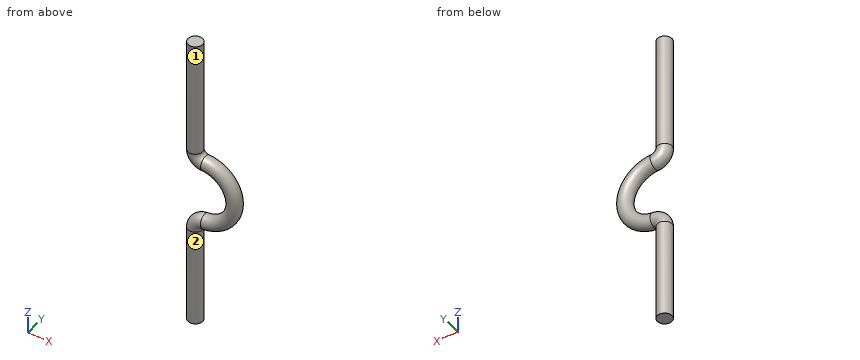
from build123d import *

# Parameters (mm, degrees)
CROQUIS2_R = 3.5


with BuildPart() as part:
    # Barrer2: sweep along a path in Croquis1
    with BuildLine(Plane(origin=(0, 0, 0), x_dir=(1, 0, 0), z_dir=(0, 1, 0))) as barrer2_path:
        Line((0, 0), (0, 55.031280577))
        ThreePointArc((0, 55.031280577), (1.355655066, 58.454546562), (4.6875, 60.021505397))
        ThreePointArc((4.6875, 60.021505397), (18.75, 74.992179856), (4.6875, 89.962854314))
        ThreePointArc((4.6875, 89.962854314), (1.355655066, 91.52981315), (0, 94.953079134))
        Line((0, 94.953079134), (0, 142))
    # Croquis2 → Barrer2 (sweep)
    with BuildSketch(Plane.XY):
        Circle(CROQUIS2_R)
    sweep(path=barrer2_path.line)


solid = part.part
Build history of the part. All positions in model axes, mm. Face numbers are marked on the shaded views. A direction names the side the tool comes from. Round coordinates to 2 decimals unless told otherwise and drop trailing zeros. Write each loop counter-clockwise with the first axis right and the second up, starting at its lowest first coordinate (ties: lowest second). Pieces come first, ordered by that corner, then holes. Notation, with made-up numbers: (40, 27.25) -> (46, 27.25) arc R17 ccw to (46, 60.25) -> close; hole circle Ø7 at (57.5, 48). An arc over 180 degrees is marked (long way). Use one line per item in the form item = value.
Q1. Drop flat-ended pins along their axis: P1, Ø1, axis at x = 5, y = -2, coming from the +Z side; P2, Ø3, axis at x = 12, y = -1.5, coming from the +Z side; P3, Ø1.5, axis at x = 15, y = 0.5, coming from the +Z side. Give the stop position or say it passes through.
Conclusion:
P1 = -56.87
P2 = -57.94
P3 = -59.79
Q2. Tool access for the marked faces 1 and 2: list every direction of +Z, -Z, +X, -X, +Y, -Y with a clear straight run to the whole face (end or side of a thin tool).
Conclusion:
face_1 = +Z
face_2 = -Z
Q3. Band-saw the part on A-A, the plane y = 0. Write the cut outline in (x, z).
Conclusion:
outline = (-3.5, -142) -> (3.5, -142) -> (3.5, -94.95) arc R1.5 cw to (4.91, -93.46) arc R18.5 ccw to (4.91, -56.53) arc R1.5 cw to (3.5, -55.03) -> (3.5, 0) -> (-3.5, 0) -> (-3.5, -55.03) arc R8.5 ccw to (4.47, -63.51) arc R11.5 cw to (4.47, -86.47) arc R8.5 ccw to (-3.5, -94.95) -> close
Q4. Band-saw the part on B-B, the plane z = -24.5. Write the cut outline in (x, y).
Conclusion:
outline = circle Ø7 at (0, 0)
Q5. Drill centre lines: L1, parallel to X at y = 0, z = -108.5; L2, parallel to Z at x = -1.5, y = 0.5. Where is each one in solid material? Low to high.
Conclusion:
L1 = -3.5 to 3.5
L2 = -142 to -89.53, -60.45 to 0
